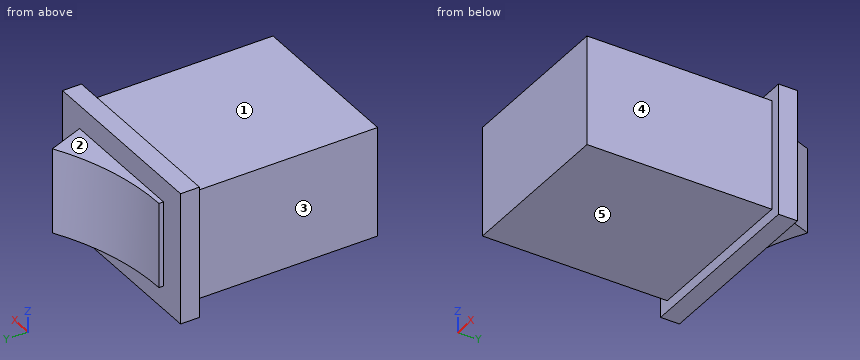
from build123d import *

# Parameters (mm, degrees)
SKETCH1_W                = 18.4
SKETCH1_H                = 20.57
BOSS_EXTRUDE1_DEPTH      = 6.125
BOSS_EXTRUDE1_DEPTH_BACK = 6.125
SKETCH1_3_W              = 20.75
SKETCH1_3_H              = 2.1
BOSS_EXTRUDE2_DEPTH      = 7.35
BOSS_EXTRUDE2_DEPTH_BACK = 7.35
BOSS_EXTRUDE3_DEPTH      = 4.75
BOSS_EXTRUDE3_DEPTH_BACK = 4.75


with BuildPart() as part:
    # Sketch1 → Boss-Extrude1 (new body, two sides)
    with BuildSketch(Plane.XY) as boss_extrude1_sk:
        Rectangle(SKETCH1_W, SKETCH1_H)
    extrude(amount=BOSS_EXTRUDE1_DEPTH)
    extrude(boss_extrude1_sk.sketch, amount=-BOSS_EXTRUDE1_DEPTH_BACK)

    # Sketch1_3 → Boss-Extrude2 (add, two sides)
    with BuildSketch(Plane.XY) as boss_extrude2_sk:
        with Locations((0, 11.335)):
            Rectangle(SKETCH1_3_W, SKETCH1_3_H)
    extrude(amount=BOSS_EXTRUDE2_DEPTH)
    extrude(boss_extrude2_sk.sketch, amount=-BOSS_EXTRUDE2_DEPTH_BACK)

    # Sketch1_4 → Boss-Extrude3 (add, two sides)
    with BuildSketch(Plane.XY) as boss_extrude3_sk:
        with BuildLine():
            Line((-7.375, 12.885), (-7.375, 12.385))
            Line((-7.375, 12.385), (7.375, 12.385))
            Line((7.375, 12.385), (5.840957819, 16.385))
            ThreePointArc((5.840957819, 16.385), (-0.539220215, 13.77482664), (-7.375, 12.885))
        make_face()
    extrude(amount=BOSS_EXTRUDE3_DEPTH)
    extrude(boss_extrude3_sk.sketch, amount=-BOSS_EXTRUDE3_DEPTH_BACK)


solid = part.part
Source: CAD feature listing. Evaluate the final solid. Frame: model axes, mm. Face numbers are marked on the shaded views. A direction names the side the tool comes from. Coordinates: 2 decimals unless noted, no trailing zeros. Loops run counter-clockwise (first coordinate to the right, second up) from the corner with the lowest first, then second, coordinate; pieces in that order, holes last. Notation, with made-up numbers: (70.5, 16) - (120.5, 16) arc R18 ccw to (120.5, 44) - close; hole circle Ø10 at (51.5, -4). An arc over 180 degrees is marked (long way). One line per item, written item: value. Start each with the question number.
1. Set-up query: the marked faces 1, 2, 3, 4 and 5. Return all of +Z, -Z, +X, -X, +Y, -Y with unobstructed straight access to the full face (end or side cutting, diameter ignored); none if empty.
2. Section A-A (z = 1.25). Return the cut outline in (x, y) (3 decimals), and give its area (3 significant figures).
3. Ray query, L1, parallel to X at y = 6.5, z = 5; L2, parallel to Z at x = 3.5, y = 13; L3, parallel to Z at x = 3.5, y = -5.25 (3 decimals). Return the intervals inside material, ascending.
4. Section C-C (y = 8.25). Return the cut outline in (x, z) (3 decimals), and give its area (3 significant figures).
5. Section B-B (x = -5). Return the cut outline in (y, z) (3 decimals).
6. Contact query for flat-ended pins moving along their axis: P1, Ø5, axis at x = -1.5, z = -5, coming from the +Y side; P2, Ø1, axis at x = -4.5, y = 1, coming from the -Z side (3 decimals); P3, Ø1, axis at x = -1.5, y = -4.5, coming from the +Z side (3 decimals); P4, Ø6, axis at x = -1, y = 9.5, coming from the +Z side. Output: stop coordinate, or through.
Verdict:
1. face 1: +Z, +X, -X, -Y
1. face 2: +Z, +X, -X, +Y
1. face 3: +Z, -Z, -X, -Y
1. face 4: +Z, -Z, +X, -Y
1. face 5: -Z, +X, -X, -Y
2. outline: (-10.375, 10.285) - (-9.2, 10.285) - (-9.2, -10.285) - (9.2, -10.285) - (9.2, 10.285) - (10.375, 10.285) - (10.375, 12.385) - (7.375, 12.385) - (5.841, 16.385) arc R26.702 cw to (-7.375, 12.885) - (-7.375, 12.385) - (-10.375, 12.385) - close
2. area: 447 mm2
3. L1: x = -9.2 to 9.2
3. L2: z = -4.75 to 4.75
3. L3: z = -6.125 to 6.125
4. outline: (-9.2, -6.125) - (9.2, -6.125) - (9.2, 6.125) - (-9.2, 6.125) - close
4. area: 225 mm2
5. outline: (-10.285, -6.125) - (10.285, -6.125) - (10.285, -7.35) - (12.385, -7.35) - (12.385, -4.75) - (12.991, -4.75) - (12.991, 4.75) - (12.385, 4.75) - (12.385, 7.35) - (10.285, 7.35) - (10.285, 6.125) - (-10.285, 6.125) - close
6. P1: stops at y = 14.23
6. P2: stops at z = -6.125
6. P3: stops at z = 6.125
6. P4: stops at z = 7.35
